For this review, use the dimensioned drawing (mm, ordinates from the lowest corner) and the shaded views. Round coordinates to 2 decimals unless told otherwise and drop trailing zeros. Loops run counter-clockwise (first coordinate to the right, second up) from the corner with the lowest first, then second, coordinate; pieces in that order, holes last. Notation, with made-up numbers: (30.5, 89.5) - (43.5, 89.5) arc R7 cw to (43.5, 98.5) - close; hole circle Ø7 at (-1, 66.5). An arc over 180 degrees is marked (long way). Answer as CSV lines item,"result". Start each with the question number.
(1) Consider section A-A (x = 228). Give the boundary of the cut face in (y, z) (1 decimal), and give its area (3 significant figures).
(2) Consider section C-C (x = 25). Give the boundary of the cut face in (y, z), and give its area (3 significant figures).
(3) For P1, Ø23, axis at x = 229.08, z = 231.41, coming from the +Y side, flat-tipped, find the tip position at first contact; note if it passes through.
(4) Wall thickness on L1, parallel to X at y = 2, z = 23; L2, parallel to Z at x = 19, y = 1 (1 decimal); L3, parallel to X at y = 0.5, z = 26 (1 decimal): over which ranges is each line inside the solid? List them lowest first.
(5) Consider section B-B (y = 8). Give the boundary of the cut face in (x, z), and give its area (3 significant figures).
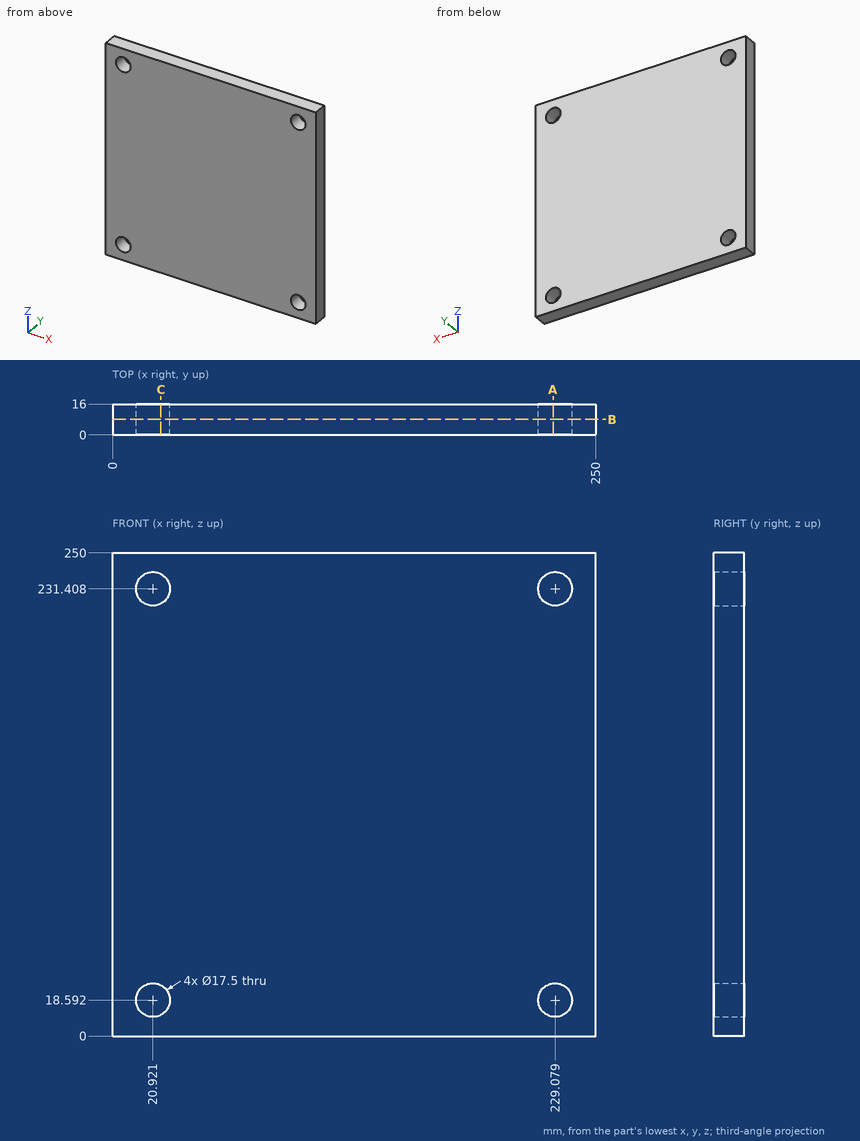
Determined:
1,outline,"(0, 0) - (16, 0) - (16, 9.9) - (0, 9.9) - close; (0, 27.3) - (16, 27.3) - (16, 222.7) - (0, 222.7) - close; (0, 240.1) - (16, 240.1) - (16, 250) - (0, 250) - close"
1,area,"3,440 mm^2"
2,outline,"(0, 0) - (16, 0) - (16, 10.85) - (0, 10.85) - close; (0, 26.33) - (16, 26.33) - (16, 223.67) - (0, 223.67) - close; (0, 239.15) - (16, 239.15) - (16, 250) - (0, 250) - close"
2,area,"3,500 mm^2"
3,P1,"stops at y = 16"
4,L1,"x = 0 to 13.36, 28.48 to 221.52, 236.64 to 250"
4,L2,"z = 0 to 10.1, 27.1 to 222.9, 239.9 to 250"
4,L3,"x = 0 to 16.3, 25.6 to 224.4, 233.7 to 250"
5,outline,"(0, 0) - (250, 0) - (250, 250) - (0, 250) - close; hole circle Ø17.5 at (20.92, 18.59); hole circle Ø17.5 at (20.92, 231.41); hole circle Ø17.5 at (229.08, 18.59); hole circle Ø17.5 at (229.08, 231.41)"
5,area,"61,500 mm^2"
